Design review of the part built by this model. Coordinates are the model's own, in mm. Face numbers are marked on the shaded views. A direction names the side the tool comes from. Give positions to 0.01 mm unless a question says otherwise; leave off trailing zeros. Order: outer loops, then holes, each group sorted by start corner. A loop starts at its lowest first (then second) coordinate and runs counter-clockwise, first axis right, second up. Notation, with made-up numbers: (19, 48.25) -> (67, 48.25) arc R26 cw to (67, 72.25) -> close; hole circle Ø11 at (-12.5, -3). An arc over 180 degrees is marked (long way). Return JSON: item names as keys, results as strings.
Autodesk Inventor part; units mm, degrees
ref_plane "Work Plane1" through (0, 0, 0) normal (0, 1, 0) x (0, 0, 1)
ref_plane "YZ Plane" through (0, 0, 0) normal (1, 0, 0) x (0, 1, 0)
ref_plane "XZ Plane" through (0, 0, 0) normal (0, 1, 0) x (-1, 0, 0)
sketch "Sketch1" plane through (0, 0, 0) normal (0, 0, 1) x (1, 0, 0)
  line L0 (0, 0) -> (-20.7182, 20.7182) construction
  line L1 (7.0711, 0) -> (29.3, 0) construction
  line L2 (0, 0) -> (20.7182, 20.7182) construction
  line L3 (0, 0) -> (29.3, 0) construction
  line L4 (-20.7182, 20.7182) -> (20.7182, 20.7182) construction
  circle A0 centre (-20.7182, 20.7182) radius 2.5
  circle A1 centre (20.7182, 20.7182) radius 2.5
  circle A2 centre (-20.7182, -20.7182) radius 2.5
  circle A3 centre (20.7182, -20.7182) radius 2.5
  arc A4 (-24.2538, -17.1827) -> (-17.1827, -24.2538) centre (-20.7182, -20.7182) ccw
  line L5 (20.7182, 20.7182) -> (13.788, 27.6485) construction
  arc A5 (24.2538, 17.1827) -> (17.1827, 24.2538) centre (20.7182, 20.7182) ccw
  arc A6 (-17.1827, 24.2538) -> (-24.2538, 17.1827) centre (-20.7182, 20.7182) ccw
  arc A7 (17.1827, -24.2538) -> (24.2538, -17.1827) centre (20.7182, -20.7182) ccw
  line L6 (17.1827, 24.2538) -> (0, 7.0711)
  line L7 (-7.0711, 0) -> (-24.2538, -17.1827)
  line L8 (24.2538, -17.1827) -> (7.0711, 0)
  line L9 (0, 7.0711) -> (-17.1827, 24.2538)
  line L10 (24.2538, 17.1827) -> (7.0711, 0)
  line L11 (0, -7.0711) -> (-17.1827, -24.2538)
  line L12 (17.1827, -24.2538) -> (0, -7.0711)
  line L13 (-7.0711, 0) -> (-24.2538, 17.1827)
  dimension "d0" = 29.3
  dimension "d1" = 135
  dimension "d2" = 29.3
  dimension "d3" = 45
  dimension "d4" = 2.5
  dimension "d5" = 2.5
  dimension "d6" = 5
  dimension "d7" = 5
extrude "Extrusion1" add sketch "Sketch1" along normal blind 4
sketch "Sketch2" plane through (0, 0, 4) normal (0, 0, 1) x (1, 0, 0)
  circle A0 centre (0, 0) radius 25.01
  dimension "d10" = 25.01
extrude "Extrusion2" add sketch "Sketch2" along normal blind 50
chamfer "Chamfer1" distance 4 angle 45 4 edges at (23.9509, 7.201, 4) (0, -25.01, 4) (-25.01, 0, 4) (0, 25.01, 4)
sketch "Sketch3" plane through (0, 0, 54) normal (0, 0, 1) x (1, 0, 0)
  line L0 (0, 0) -> (25.01, 0)
  circle A0 centre (0, 0) radius 25.01
sketch "Sketch4" plane through (0, 0, 0) normal (0, 0, -1) x (-1, 0, 0)
  point P0 (0, 0)
  point P1 (0, 0)
ref_plane "Work Plane1" through (0, 0, 0) normal (0, 1, 0) x (0, 0, 1)
sketch "Sketch5" plane through (0, 0, 0) normal (0, 1, 0) x (0, 0, 1)
  line L0 (54, -25.01) -> (54, 25.01)
  line L1 (54, 0) -> (79, 0)
  line L2 (79, 0) -> (79, 3)
  line L3 (79, 3) -> (64, 3)
  line L4 (64, 3) -> (64, 8)
  line L5 (64, 8) -> (60.25, 8)
  line L6 (60.25, 8) -> (60.25, 16)
  line L7 (60.25, 16) -> (54, 25.01)
  point P0 (0, 0)
  dimension "d16" = 25
  dimension "d17" = 3
  dimension "d18" = 15
  dimension "d19" = 5
  dimension "d20" = 3.75
  dimension "d21" = 8
revolve "Revolution1" add sketch "Sketch5" angle 360 about axis through (0, 0, 54) along (0, 0, 1)
properties part number "Motor Turnigy G60 500kv"
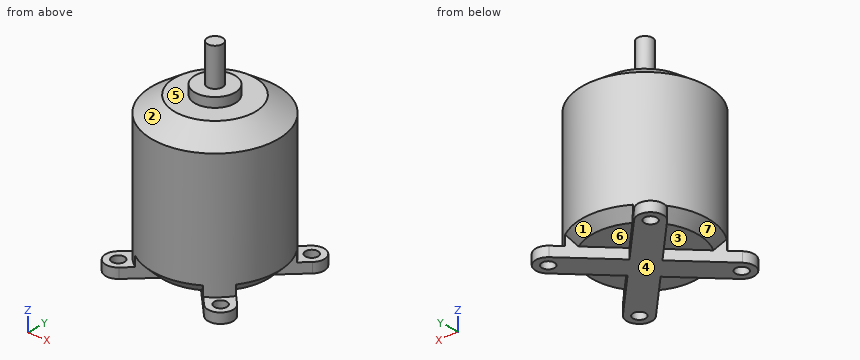
Item 1: Mouldability with a two-part tool opening along Y and no side actions: class the marked faces 1, 2, 3 and 4 as released by +Y, released by -Y, zero draft, split by the parting line, or undercut.
Result set:
{"face 1": "released by +Y", "face 2": "split by the parting line", "face 3": "undercut", "face 4": "zero draft"}
Item 2: For pin 1 (11 mm diameter, centred on x = 15.5, y = 0, fed in from -Z); pin 2 (6 mm diameter, centred on y = 9.5, z = 41, fed in from +X); pin 3 (5 mm diameter, centred on x = 3, y = -8.5, fed in from +Z); pin 4 (3 mm diameter, centred on x = 20.72, y = -20.72, fed in from -Z), all flat-tipped, find the tip position at first contact; note any pin that passes through.
Result set:
{"pin 1": "stops at z = 4", "pin 2": "stops at x = 24.15", "pin 3": "stops at z = 64", "pin 4": "passes through"}
Item 3: Add section A-A (z = 25.5). Give the boundary of the cut face in (x, y), plus the area to 3 significant figures.
Result set:
{"outline": "circle Ø50.02 at (0, 0)", "area": "1,970 mm^2"}
Item 4: Machinability: for the marked faces 5, 6 and 7, which of the approach directions +Z, -Z, +X, -X, +Y, -Y give a long, thin tool a straight path to every point of the face, cutting with its end or side? Answer none if there is none.
Result set:
{"face 5": "+Z", "face 6": "-Z, +Y", "face 7": "-Z, -X"}
Item 5: Wall thickness on L1, parallel to Z at x = -7, y = 2.5; L2, parallel to Z at x = 18, y = 18; L3, parallel to Y at x = 14, z = 51: over which ranges is each line inside the solid? List them lowest first. Write a range as [from, to].
Result set:
{"L1": "z = [0, 64]", "L2": "z = [0, 4]", "L3": "y = [-20.72, 20.72]"}
